Verification items for the finished model (mm, model axes). A direction names the side the tool comes from. Give positions to 0.01 mm unless a question says otherwise; leave off trailing zeros. Write each loop counter-clockwise with the first axis right and the second up, starting at its lowest first coordinate (ties: lowest second). Pieces come first, ordered by that corner, then holes.
from build123d import *

# Parameters (mm, degrees)
SKETCH1_W           = 150
SKETCH1_H           = 129.788
BOSS_EXTRUDE1_DEPTH = 5
SKETCH1_3_W         = 60
SKETCH1_3_H         = 6
BOSS_EXTRUDE2_DEPTH = 15
FILLET1_R           = 1


with BuildPart() as part:
    # Sketch1 → Boss-Extrude1 (new body)
    with BuildSketch(Plane(origin=(0, 0, 0), x_dir=(1, 0, 0), z_dir=(0, 1, 0))):
        with Locations((0, -1.75)):
            Rectangle(SKETCH1_W, SKETCH1_H)
    extrude(amount=BOSS_EXTRUDE1_DEPTH)

    # Sketch1_3 → Boss-Extrude2 (add)
    with BuildSketch(Plane(origin=(0, 0, 0), x_dir=(1, 0, 0), z_dir=(0, 1, 0))):
        with Locations((-45, 60.144)):
            Rectangle(SKETCH1_3_W, SKETCH1_3_H)
        with Locations((-45, 40.096)):
            Rectangle(SKETCH1_3_W, SKETCH1_3_H)
        with Locations((-45, 20.048)):
            Rectangle(SKETCH1_3_W, SKETCH1_3_H)
        with Locations((-45, 0)):
            Rectangle(SKETCH1_3_W, SKETCH1_3_H)
        with Locations((45, 56.644)):
            Rectangle(SKETCH1_3_W, SKETCH1_3_H)
        with Locations((45, 36.596)):
            Rectangle(SKETCH1_3_W, SKETCH1_3_H)
        with Locations((45, 16.548)):
            Rectangle(SKETCH1_3_W, SKETCH1_3_H)
        with Locations((45, -3.5)):
            Rectangle(SKETCH1_3_W, SKETCH1_3_H)
        with Locations((-45, -20.048)):
            Rectangle(SKETCH1_3_W, SKETCH1_3_H)
        with Locations((-45, -40.096)):
            Rectangle(SKETCH1_3_W, SKETCH1_3_H)
        with Locations((-45, -60.144)):
            Rectangle(SKETCH1_3_W, SKETCH1_3_H)
        with Locations((45, -23.548)):
            Rectangle(SKETCH1_3_W, SKETCH1_3_H)
        with Locations((45, -43.596)):
            Rectangle(SKETCH1_3_W, SKETCH1_3_H)
        with Locations((45, -63.644)):
            Rectangle(SKETCH1_3_W, SKETCH1_3_H)
    extrude(amount=BOSS_EXTRUDE2_DEPTH)

    # Fillet1
    fillet1_edges = [part.edges().sort_by_distance(p)[0] for p in [
        (-15, 10, -3),
        (-75, 10, -3),
        (-75, 10, 3),
        (-15, 10, 3),
        (-15, 10, -23.048),
        (-75, 10, -23.048),
        (-75, 10, -17.048),
        (-15, 10, -17.048),
        (75, 2.5, -63.144),
        (75, 7.5, 66.644),
        (-75, 2.5, 66.644),
        (-75, 7.5, -63.144),
        (-15, 10, -43.096),
        (-75, 10, -43.096),
        (-75, 10, -37.096),
        (-15, 10, -37.096),
        (-75, 10, -57.144),
        (-15, 10, -57.144),
        (-15, 10, -63.144),
        (75, 10, -59.644),
        (15, 10, -59.644),
        (15, 10, -53.644),
        (75, 10, -53.644),
        (75, 10, -39.596),
        (15, 10, -39.596),
        (15, 10, -33.596),
        (75, 10, -33.596),
        (75, 10, -19.548),
        (15, 10, -19.548),
        (15, 10, -13.548),
        (75, 10, -13.548),
        (75, 10, 0.5),
        (15, 10, 0.5),
        (15, 10, 6.5),
        (75, 10, 6.5),
        (75, 10, 20.548),
        (15, 10, 20.548),
        (15, 10, 26.548),
        (75, 10, 26.548),
        (75, 10, 40.596),
        (15, 10, 40.596),
        (15, 10, 46.596),
        (75, 10, 46.596),
        (75, 10, 60.644),
        (15, 10, 60.644),
        (15, 10, 66.644),
        (-15, 10, 57.144),
        (-75, 10, 57.144),
        (-75, 10, 63.144),
        (-15, 10, 63.144),
        (-15, 10, 37.096),
        (-75, 10, 37.096),
        (-75, 10, 43.096),
        (-15, 10, 43.096),
        (-15, 10, 17.048),
        (-75, 10, 17.048),
        (-75, 10, 23.048),
        (-15, 10, 23.048),
    ]]
    fillet(fillet1_edges, radius=FILLET1_R)


solid = part.part
Item 1: Sectioned sample at C-C on z = -47.5. Record the cut outline in (x, y).
Answer key:
outline: (-75, 0) - (75, 0) - (75, 5) - (-75, 5) - close
Item 2: Scan lines: line 1 along Y through (x, z) = (68, -27); line 2 along X through (y, z) = (8.25, 42); line 3 along X through (y, z) = (7.5, 39). Record each from-to range of solid material in increasing order.
Answer key:
line 1: y = 0 to 5
line 2: x = -75 to -15, 15 to 75
line 3: x = -75 to -15
Item 3: Release check for a two-part mould opening along Z. For faces 4 (the face through (45, 10, -13.548)), 5 (the face through (45, 10, -59.644)), 6 (the face through (-45, 15, -40)) record: released by +Z, released by -Z, zero draft, split by the parting line, or undercut.
Answer key:
face 4: undercut
face 5: released by -Z
face 6: zero draft
Item 4: Sectioned sample at A-A on y = 8. State how many separate pieces and enclosed holes the cut face has, then the cut area to 3 significant figures.
Answer key:
separate pieces: 14
enclosed holes: 0
area: 5,030 mm2
Item 5: Sectioned sample at D-D on x = 6. Record the cut outline in (y, z), then the cut area to 3 significant figures.
Answer key:
outline: (0, -63.14) - (5, -63.14) - (5, 66.64) - (0, 66.64) - close
area: 649 mm2
Item 6: Depth check by flat-ended pin: pin 1 (2 mm diameter, centred on x = -37.5, y = 7, fed in from +Z); pin 2 (6 mm diameter, centred on x = 48.5, z = -15, fed in from -Y); pin 3 (8 mm diameter, centred on x = 52.5, y = 10, fed in from -Z); pin 4 (5 mm diameter, centred on x = 50, z = 36.5, fed in from +Y). Enter the tip coordinate at first touch or a pass-through.
Answer key:
pin 1: stops at z = 63.14
pin 2: stops at y = 0
pin 3: stops at z = -59.64
pin 4: stops at y = 5
Item 7: Set-up check for faces 1 (the face through (45, 10, 60.644)), 2 (the face through (-45, 10, -23.048)), 3 (the face through (-15, 10, 40)): record each of +Z, -Z, +X, -X, +Y, -Y from which the full face is reachable in a straight line by a thin tool's end or side.
Answer key:
face 1: +X, +Y
face 2: +X, -X, +Y
face 3: +Z, -Z, +Y
